from build123d import *

# Parameters (mm, degrees)
SKETCH007_R      = 1.5
EXTRUDE012_DEPTH = 75
SKETCH008_R      = 13
EXTRUDE014_DEPTH = 3.5
EXTRUDE002_DEPTH = 44
SKETCH002_W      = 3.5
SKETCH002_H      = 8
EXTRUDE003_DEPTH = 75
SKETCH003_W      = 40
SKETCH003_H      = 10
EXTRUDE005_DEPTH = 30
SKETCH004_W      = 68.5
SKETCH004_H      = 30
EXTRUDE006_DEPTH = 6
SKETCH005_W      = 5.5
SKETCH005_H      = 24
EXTRUDE008_DEPTH = 12
EXTRUDE009_DEPTH = 3
EXTRUDE010_DEPTH = 3
EXTRUDE_DEPTH    = 9
EXTRUDE017_DEPTH = 20
EXTRUDE015_DEPTH = 60
FILLET_R         = 15
FILLET001_R      = 14
FILLET002_R      = 5
CHAMFER_SIZE     = 10


with BuildPart() as extrude012:
    # Sketch007 → Extrude012 (new body)
    with BuildSketch(Plane.XY):
        with Locations((-45, 23)):
            Circle(SKETCH007_R)
        with Locations((45, 23)):
            Circle(SKETCH007_R)
    extrude(amount=EXTRUDE012_DEPTH)


with BuildPart() as extrude014:
    # Sketch008 → Extrude014 (new body)
    with BuildSketch(Plane.XY):
        with Locations((-45, 23)):
            Circle(SKETCH008_R)
        with Locations((45, 23)):
            Circle(SKETCH008_R)
    extrude(amount=EXTRUDE014_DEPTH)


with BuildPart() as extrude002:
    # Sketch001 (on Face6 of Extrude) → Extrude002 (new body)
    with BuildSketch(Plane.XY.offset(9)):
        with BuildLine():
            Line((-14, 21), (-14, -1))
            ThreePointArc((-14, -1), (-10.485281, -9.485281), (-2, -13))
            Line((-2, -13), (2, -13))
            ThreePointArc((2, -13), (10.485281, -9.485281), (14, -1))
            Line((14, 21), (14, -1))
            Line((-14, 21), (14, 21))
        make_face()
    extrude(amount=EXTRUDE002_DEPTH)


with BuildPart() as extrude003:
    # Sketch002 (on Face6 of Extrude) → Extrude003 (new body)
    with BuildSketch(Plane.XY.offset(9)):
        with Locations((-17.75, 7)):
            Rectangle(SKETCH002_W, SKETCH002_H)
        with Locations((17.75, 7)):
            Rectangle(SKETCH002_W, SKETCH002_H)
    extrude(amount=EXTRUDE003_DEPTH)


with BuildPart() as extrude005:
    # Sketch003 (on Face6 of Extrude) → Extrude005 (new body)
    with BuildSketch(Plane.XY.offset(9)):
        with Locations((0, 7)):
            Rectangle(SKETCH003_W, SKETCH003_H)
    extrude(amount=EXTRUDE005_DEPTH)


with BuildPart() as extrude006:
    # Sketch004 → Extrude006 (new body)
    with BuildSketch(Plane.XY):
        with Locations((0, 24)):
            Rectangle(SKETCH004_W, SKETCH004_H)
    extrude(amount=EXTRUDE006_DEPTH)


with BuildPart() as extrude008:
    # Sketch005 (on Face6 of Extrude) → Extrude008 (new body)
    with BuildSketch(Plane.XY.offset(9)):
        with Locations((-2.75, 12)):
            Rectangle(SKETCH005_W, SKETCH005_H)
    extrude(amount=EXTRUDE008_DEPTH)


with BuildPart() as extrude009:
    # Sketch006 → Extrude009 (new body)
    with BuildSketch(Plane.XY):
        with BuildLine():
            ThreePointArc((-23.5, 92), (-27.742641, 90.242641), (-29.5, 86))
            Line((-29.5, 48), (-29.5, 86))
            ThreePointArc((-29.5, 48), (-27.742641, 43.757359), (-23.5, 42))
            Line((23.5, 42), (-23.5, 42))
            ThreePointArc((23.5, 42), (27.742641, 43.757359), (29.5, 48))
            Line((29.5, 86), (29.5, 48))
            ThreePointArc((29.5, 86), (27.742641, 90.242641), (23.5, 92))
            Line((-23.5, 92), (23.5, 92))
        make_face()
    extrude(amount=EXTRUDE009_DEPTH)


with BuildPart() as extrude010:
    # Sketch006 → Extrude010 (new body)
    with BuildSketch(Plane.XY):
        with BuildLine():
            ThreePointArc((-23.5, 92), (-27.742641, 90.242641), (-29.5, 86))
            Line((-29.5, 48), (-29.5, 86))
            ThreePointArc((-29.5, 48), (-27.742641, 43.757359), (-23.5, 42))
            Line((23.5, 42), (-23.5, 42))
            ThreePointArc((23.5, 42), (27.742641, 43.757359), (29.5, 48))
            Line((29.5, 86), (29.5, 48))
            ThreePointArc((29.5, 86), (27.742641, 90.242641), (23.5, 92))
            Line((-23.5, 92), (23.5, 92))
        make_face()
    extrude(amount=EXTRUDE010_DEPTH)


with BuildPart() as fusion001:
    # Sketch → Extrude (new body)
    with BuildSketch(Plane.XY):
        with BuildLine():
            ThreePointArc((-31.25, -1), (0, -13), (31.25, -1))
            Line((31.25, -1), (31.25, 47.5))
            Line((-31.25, 47.5), (31.25, 47.5))
            Line((-31.25, -1), (-31.25, 47.5))
        make_face()
    extrude(amount=EXTRUDE_DEPTH)

    # Fusion: union Extrude002, Extrude003, Extrude005, Extrude006, Extrude008, Extrude009, Extrude010
    add(extrude002.part)
    add(extrude003.part)
    add(extrude005.part)
    add(extrude006.part)
    add(extrude008.part)
    add(extrude009.part)
    add(extrude010.part)

    # Fusion001: union Extrude012, Extrude014
    add(extrude012.part)
    add(extrude014.part)


with BuildPart() as extrude017:
    # Sketch010 → Extrude017 (new body)
    with BuildSketch(Plane.XY):
        with BuildLine():
            ThreePointArc((-45, 38), (-60, 23), (-45, 8))
            Line((-45, 8), (45, 8))
            ThreePointArc((45, 8), (60, 23), (45, 38))
            Line((45, 38), (-45, 38))
        make_face()
    extrude(amount=EXTRUDE017_DEPTH)


with BuildPart() as cut:
    # Sketch009 → Extrude015 (new body)
    with BuildSketch(Plane.XY):
        with BuildLine():
            Line((-37.5, 99), (-37.5, -13))
            ThreePointArc((-37.5, -13), (0, -33), (37.5, -13))
            Line((37.5, 99), (37.5, -13))
            Line((-37.5, 99), (37.5, 99))
        make_face()
    extrude(amount=EXTRUDE015_DEPTH)

    # Fusion002: union Extrude017
    add(extrude017.part)

    # Fillet
    fillet_edges = [cut.edges().sort_by_distance(p)[0] for p in [
        (-37.5, -13, 30),
        (-37.5, 99, 30),
        (37.5, -13, 30),
        (37.5, 99, 30),
    ]]
    fillet(fillet_edges, radius=FILLET_R)

    # Fillet001
    fillet001_edges = [cut.edges().sort_by_distance(p)[0] for p in [
        (-41.25, 38, 20),
        (-41.25, 8, 20),
        (-60, 23, 20),
        (41.25, 38, 20),
        (60, 23, 20),
        (41.25, 8, 20),
    ]]
    fillet(fillet001_edges, radius=FILLET001_R)

    # Fillet002
    fillet002_edges = [cut.edges().sort_by_distance(p)[0] for p in [
        (-37.5, 8, 3),
        (-37.5, 12.100505, 15.899495),
        (-37.5, 23, 20),
        (-37.5, 33.899495, 15.899495),
        (-37.5, 38, 3),
        (37.5, 8, 3),
        (37.5, 12.100505, 15.899495),
        (37.5, 23, 20),
        (37.5, 33.899495, 15.899495),
        (37.5, 38, 3),
    ]]
    fillet(fillet002_edges, radius=FILLET002_R)

    # Chamfer
    chamfer_edges = [cut.edges().sort_by_distance(p)[0] for p in [
        (-37.5, 38.038835, 60),
        (-33.106602, 94.606602, 60),
        (-36.515628, -13.26669, 60),
        (0, -33, 60),
        (36.515628, -13.26669, 60),
        (37.5, 38.038835, 60),
        (33.106602, 94.606602, 60),
        (0, 99, 60),
    ]]
    chamfer(chamfer_edges, length=CHAMFER_SIZE)

    # Cut: cut Fusion001
    add(fusion001.part, mode=Mode.SUBTRACT)


solid = cut.part
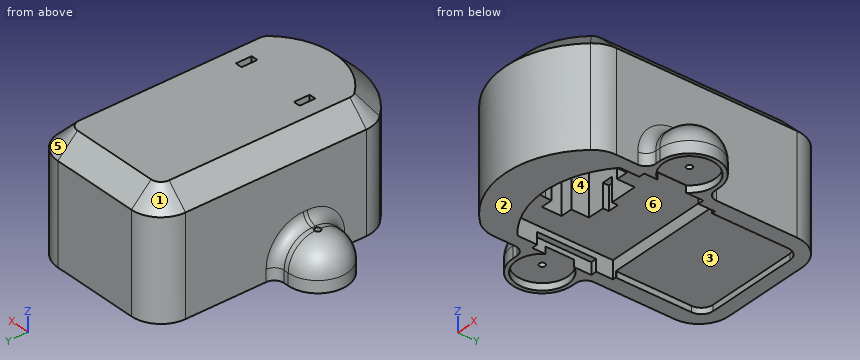
Build history of the part. All positions in model axes, mm. Face numbers are marked on the shaded views. A direction names the side the tool comes from. Round coordinates to 2 decimals unless told otherwise and drop trailing zeros. Write each loop counter-clockwise with the first axis right and the second up, starting at its lowest first coordinate (ties: lowest second). Pieces come first, ordered by that corner, then holes. Notation, with made-up numbers: (-28.75, 75) - (-8.75, 75) arc R23 ccw to (-8.75, 103) - close; hole circle Ø2 at (39, 49). An arc over 180 degrees is marked (long way). Use CSV: the item, a comma, the result in double quotes.
(1) Wall check: line 1 (Y direction, x = -45, z = 2.4); line 2 (Y direction, x = 1.5, z = 32.5); line 3 (X direction, y = 6, z = 41.5). Give the ranges that are in metal, low to high.
Response:
line 1,"8 to 10, 36 to 38"
line 2,"-32.98 to -13, 21 to 99"
line 3,"-37.5 to -19.5, -16 to -14, 14 to 16, 19.5 to 37.5"
(2) Band-saw the part on B-B (y = 69). Write the cut outline in (x, z), plus the area to 3 significant figures.
Response:
outline,"(-37.5, 0) - (-29.5, 0) - (-29.5, 3) - (29.5, 3) - (29.5, 0) - (37.5, 0) - (37.5, 50) - (27.5, 60) - (-27.5, 60) - (-37.5, 50) - close"
area,"4,220 mm²"
(3) Mould opens along Y. For the marked faces 1, 2, 3 and 4 say: pulls with the +Y half, pulls with the -Y half, needs draft (parallel to the pull), parting line crosses it, or undercut.
Response:
face 1,"pulls with the +Y half"
face 2,"needs draft"
face 3,"undercut"
face 4,"undercut"
(4) 3-axis set-ups, long thin cutter, end or side, ignore diameter. For the marked faces 5 and 6: which of +Z, -Z, +X, -X, +Y, -Y reach the whole face in a straight line?
Response:
face 5,"+Z, +X, +Y"
face 6,"-Z"
(5) Pin check, flat tips, straight feed: P1, Ø2.5, axis at y = 17, z = 5, coming from the -X side; P2, Ø6.5, axis at y = 6, z = 50, coming from the +X side; P3, Ø3, axis at x = -16.5, z = 30, coming from the -Y side; P4, Ø1.8, axis at x = 45, y = 23, coming from the -Z side. Stop position of each tip, or through.
Response:
P1,"x = -59.23"
P2,"x = 37.5"
P3,"y = -30.44"
P4,"through"
(6) Band-saw the part on A-A (z = 55.5). Write the cut outline in (x, y), plus the area to 3 significant figures.
Response:
outline,"(-32, -7.92) arc R9.5 ccw to (-29.59, -14.25) arc R39.66 ccw to (29.59, -14.25) arc R9.5 ccw to (32, -7.92) - (32, 84) arc R9.5 ccw to (22.5, 93.5) - (-22.5, 93.5) arc R9.5 ccw to (-32, 84) - close; hole (-19.5, 3) - (-16, 3) - (-16, 11) - (-19.5, 11) - close; hole (16, 3) - (19.5, 3) - (19.5, 11) - (16, 11) - close"
area,"7,330 mm²"
(7) Band-saw the part on C-C (z = 11.5). Give the number of separate pieces and of enclosed holes in the cut face, plus the area to 3 significant figures.
Response:
separate pieces,"1"
enclosed holes,"3"
area,"9,360 mm²"
